Could you check a few things on this model? Use its own coordinates, in mm. A direction names the side the tool comes from. Round coordinates to 2 decimals unless told otherwise and drop trailing zeros. Write each loop counter-clockwise with the first axis right and the second up, starting at its lowest first coordinate (ties: lowest second). Pieces come first, ordered by that corner, then holes. Notation, with made-up numbers: (74, -5) -> (127, -5) arc R33 ccw to (127, 27) -> close; hole circle Ø4 at (79, 41). An arc over 180 degrees is marked (long way). One line per question, with ' | ' between items. Start each with the question number.
1. For faces 4 (the cylindrical face through (24.765, -21.691, 9.86)), 5 (the cylindrical face through (34.767, 12.272, 19.014)), which set-ups out of +Z, -Z, +X, -X, +Y, -Y let a thin tool reach every point of the face, with its end or its side?
2. Imagine slicing it at A-A, the plane x = -31.75. List the corners of the cut face in (y, z) for me, and give its area (3 significant figures).
3. If I drill on line 1 along X through (y, z) = (0, 18.5); line 2 along Y through (x, z) = (-31.75, 14.5); line 3 along X through (y, z) = (21.5, 8), over which ranges is the centre line in solid material (lowest first)? Write a range as [from, to].
4. Thinking about a two-plate mould opening in X: for faces 1 (the cylindrical face through (-40.324, -29.134, 10.14)), 2 (the flat face through (41.75, 0, 10)), 3 (the cylindrical face through (-24.41, -22.31, 9.86)), which applies, released by +X, released by -X, zero draft, split by the parting line, or undercut?
5. For pin 1 Ø9 at (x, y) = (-22.22, -20.64) entering from -Z; pin 2 Ø1 at (y, z) = (-10, 39) entering from +X; pin 3 Ø1.5 at (x, y) = (29, 0) entering from +Z; pin 4 Ø1.5 at (x, z) = (-12, 119) entering from +Y, each with a flat end and sliding along its axis, tell me the tip position at first contact or that it passes through.
6. Imagine slicing it at C-C, the plane z = 116. List the corners of the cut face in (x, y) for me, and give its area (3 significant figures).
7. Imagine slicing it at B-B, the plane x = 0. List the corners of the cut face in (y, z) for me, and give its area (3 significant figures).
from build123d import *

# Parameters (mm, degrees)
F0_W     = 83.5
F0_H     = 61.275
F0_R     = 2.75
F1_DEPTH = 20
F2_R     = 5
F3_R     = 12.7
F4_DEPTH = 150
F5_SIZE  = 2
F6_R     = 10
F8_DEPTH = 2


with BuildPart() as f1:
    # F0 (on Top) → F1 (new body)
    with BuildSketch(Plane.XY):
        Rectangle(F0_W, F0_H)
        with Locations((-31.75, -20.6375)):
            Circle(F0_R, mode=Mode.SUBTRACT)
        with Locations((-22.225, -20.6375)):
            Circle(F0_R, mode=Mode.SUBTRACT)
        with Locations((22.225, -20.6375)):
            Circle(F0_R, mode=Mode.SUBTRACT)
        with Locations((31.75, -20.6375)):
            Circle(F0_R, mode=Mode.SUBTRACT)
        with Locations((-31.75, 20.6375)):
            Circle(F0_R, mode=Mode.SUBTRACT)
        with Locations((-22.225, 20.6375)):
            Circle(F0_R, mode=Mode.SUBTRACT)
        with Locations((22.225, 20.6375)):
            Circle(F0_R, mode=Mode.SUBTRACT)
        with Locations((31.75, 20.6375)):
            Circle(F0_R, mode=Mode.SUBTRACT)
    extrude(amount=F1_DEPTH)

    # F2
    f2_edges = [f1.edges().sort_by_distance(p)[0] for p in [
        (-41.75, -30.6375, 10),
        (41.75, -30.6375, 10),
        (-41.75, 30.6375, 10),
        (41.75, 30.6375, 10),
    ]]
    fillet(f2_edges, radius=F2_R)

    # F3 (on Top) → F4 (join)
    with BuildSketch(Plane.XY):
        Circle(F3_R)
    extrude(amount=F4_DEPTH)

    # F5
    f5_edges = [f1.edges().sort_by_distance(p)[0] for p in [
        (-12.7, 0, 150),
    ]]
    chamfer(f5_edges, length=F5_SIZE)

    # F6
    f6_edges = [f1.edges().sort_by_distance(p)[0] for p in [
        (-12.7, 0, 20),
    ]]
    fillet(f6_edges, radius=F6_R)

    # F7 (on face) → F8 (cut)
    with BuildSketch(Plane.XY.offset(20)):
        with BuildLine():
            Line((29.793699, 2.727646), (29.793699, -0.068939))
            ThreePointArc((29.793699, -0.068939), (30.439165, -2.469058), (32.201427, -4.221665))
            Line((32.201427, -4.221665), (29.7937, -4.221665))
            Line((29.7937, -4.221665), (29.7937, -7.018251))
            ThreePointArc((29.7937, -7.018251), (34.578768, -11.803318), (39.363836, -7.018251))
            Line((39.363836, -7.018251), (39.363836, -4.221665))
            Line((39.363836, -4.221665), (36.956107, -4.221665))
            ThreePointArc((36.956107, -4.221665), (38.718369, -2.469058), (39.363835, -0.068939))
            Line((39.363835, -0.068939), (39.363835, 2.727646))
            Line((39.363835, 2.727646), (36.985549, 2.727646))
            ThreePointArc((36.985549, 2.727646), (34.578767, 12.275941), (32.171985, 2.727646))
            Line((32.171985, 2.727646), (29.793699, 2.727646))
        make_face()
    extrude(amount=-F8_DEPTH, mode=Mode.SUBTRACT)


solid = f1.part
Geometry results:
1) face 4: +Z, -Z | face 5: +Z
2) outline: (-30.64, 0) -> (-23.39, 0) -> (-23.39, 20) -> (-30.64, 20) -> close; (-17.89, 0) -> (17.89, 0) -> (17.89, 20) -> (-17.89, 20) -> close; (23.39, 0) -> (30.64, 0) -> (30.64, 20) -> (23.39, 20) -> close | area: 1,010 mm2
3) line 1: x = [-41.75, 29.79], [39.36, 41.75] | line 2: y = [-30.64, -23.39], [-17.89, 17.89], [23.39, 30.64] | line 3: x = [-41.75, -34.36], [-29.14, -24.84], [-19.61, 19.61], [24.84, 29.14], [34.36, 41.75]
4) face 1: released by -X | face 2: released by +X | face 3: undercut
5) pin 1: stops at z = 0 | pin 2: stops at x = 8.43 | pin 3: stops at z = 20 | pin 4: stops at y = 5.89
6) outline: circle Ø25.4 at (0, 0) | area: 507 mm2
7) outline: (-30.64, 0) -> (30.64, 0) -> (30.64, 20) -> (22.7, 20) arc R10 cw to (12.7, 30) -> (12.7, 148) -> (10.7, 150) -> (-10.7, 150) -> (-12.7, 148) -> (-12.7, 30) arc R10 cw to (-22.7, 20) -> (-30.64, 20) -> close | area: 4,570 mm2
